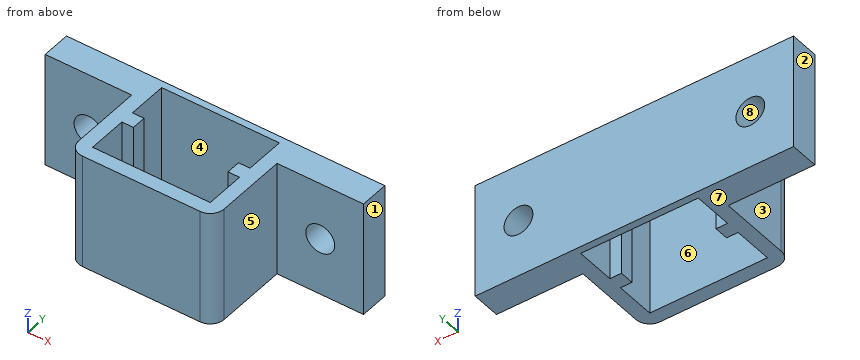
from build123d import *

# Parameters (mm, degrees)
F0_W     = 16.002
F0_H     = 12.5984
F1_DEPTH = 12.7
F2_W     = 9.525
F2_H     = 12.7
F3_DEPTH = 3.175
F4_R     = 1.524
F5_R     = 1.5875
F6_DEPTH = 25.4


with BuildPart() as f1:
    # F0 (on Top) → F1 (new body)
    with BuildSketch(Plane.XY):
        with Locations((0, 4.7752)):
            Rectangle(F0_W, F0_H)
        Polygon((6.477, 4.3688), (6.477, 0), (-6.477, 0), (-6.477, 4.3688), (-5.207, 4.3688), (-5.207, 5.9436), (-6.477, 5.9436), (-6.477, 10.3124), (6.477, 10.3124), (6.477, 5.9436), (5.207, 5.9436), (5.207, 4.3688), align=None, mode=Mode.SUBTRACT)
    extrude(amount=F1_DEPTH)

    # F2 (on face) → F3 (join)
    with BuildSketch(Plane(origin=(0, 11.0744, 0), x_dir=(-1, 0, 0), z_dir=(0, 1, 0))):
        with Locations((12.7635, 6.35)):
            Rectangle(F2_W, F2_H)
        with Locations((-12.7635, 6.35)):
            Rectangle(F2_W, F2_H)
    extrude(amount=-F3_DEPTH)

    # F4
    f4_edges = [f1.edges().sort_by_distance(p)[0] for p in [
        (-8.001, -1.524, 6.35),
        (8.001, -1.524, 6.35),
    ]]
    fillet(f4_edges, radius=F4_R)

    # F5 (on face) → F6 (cut)
    with BuildSketch(Plane.XZ.offset(-7.8994)):
        with Locations((-12.7635, 6.35)):
            Circle(F5_R)
        with Locations((12.7635, 6.35)):
            Circle(F5_R)
    extrude(amount=-F6_DEPTH, mode=Mode.SUBTRACT)


solid = f1.part
Source: CAD feature listing. Evaluate the final solid. Frame: model axes, mm. Face numbers are marked on the shaded views. A direction names the side the tool comes from. Give positions to 0.01 mm unless a question says otherwise; leave off trailing zeros. Loops run counter-clockwise (first coordinate to the right, second up) from the corner with the lowest first, then second, coordinate; pieces in that order, holes last. Notation, with made-up numbers: (69, -7.5) -> (76, -7.5) arc R25 ccw to (76, 6.5) -> close; hole circle Ø6 at (0.5, 81.5). An arc over 180 degrees is marked (long way). Use a Markdown table: item, result. Add a question column.
1) Section query C-C, the plane x = -6. Return the cut outline in (y, z), then the cut area to 3 significant figures.
2) Section query A-A, the plane z = 6.35. Count the separate pieces of the cut face and the enclosed holes in it, then the cut area to 3 significant figures.
3) Section query B-B, the plane y = 1.25. Return the cut outline in (x, z), then the cut area to 3 significant figures.
4) First-contact query: pin 1 (1.5 mm diameter, centred on y = 6, z = 10, fed in from -X); pin 2 (5 mm diameter, centred on x = 11, z = 9, fed in from -Y); pin 3 (2.5 mm diameter, centred on x = 12.76, z = 6.35, fed in from +Y); pin 4 (1.3 mm diameter, centred on y = 5.5, z = 8, fed in from +X). Flat tips, straight axial feed; report the tip coordinate or a pass-through.
5) Reachability of the marked faces 1, 2, 3, 4 and 5 from +Z, -Z, +X, -X, +Y, -Y: full face, straight path, thin tool, end or side. Return the list, or none.
6) Line query: line 1 along Y through (x, z) = (3, 2.5); line 2 along X through (y, z) = (9.75, 9.5); line 3 along X through (y, z) = (4, 8.5). Output: solid intervals per line, ascending. Write a range as [from, to].
7) Section query D-D, the plane z = 2.25. Return the cut outline in (x, y), then the cut area to 4 significant figures.
8) Pull-direction query (Z, two-part tool) for the marked faces 6, 7 and 8; classes: +Z half, -Z half, draft (parallel to the pull), parting line (faces both ways), or undercut.
Numbers:
| question | item | result |
|---|---|---|
| 1 | outline | (-1.52, 0) -> (0, 0) -> (0, 12.7) -> (-1.52, 12.7) -> close; (4.37, 0) -> (5.94, 0) -> (5.94, 12.7) -> (4.37, 12.7) -> close; (10.31, 0) -> (11.07, 0) -> (11.07, 12.7) -> (10.31, 12.7) -> close |
| 1 | area | 49.0 mm2 |
| 2 | separate pieces | 3 |
| 2 | enclosed holes | 1 |
| 2 | area | 111 mm2 |
| 3 | outline | (-8, 0) -> (-6.48, 0) -> (-6.48, 12.7) -> (-8, 12.7) -> close; (6.48, 0) -> (8, 0) -> (8, 12.7) -> (6.48, 12.7) -> close |
| 3 | area | 38.7 mm2 |
| 4 | pin 1 | stops at x = -8 |
| 4 | pin 2 | stops at y = 7.9 |
| 4 | pin 3 | passes through |
| 4 | pin 4 | stops at x = 8 |
| 5 | face 1 | +Z, -Z, +X, +Y, -Y |
| 5 | face 2 | +Z, -Z, -X, +Y, -Y |
| 5 | face 3 | +Z, -Z, -X, -Y |
| 5 | face 4 | +Z, -Z |
| 5 | face 5 | +Z, -Z, +X, -Y |
| 6 | line 1 | y = [-1.52, 0], [10.31, 11.07] |
| 6 | line 2 | x = [-17.53, -6.48], [6.48, 17.53] |
| 6 | line 3 | x = [-8, -6.48], [6.48, 8] |
| 7 | outline | (-17.53, 7.9) -> (-8, 7.9) -> (-8, 0) arc R1.52 ccw to (-6.48, -1.52) -> (6.48, -1.52) arc R1.52 ccw to (8, 0) -> (8, 7.9) -> (17.53, 7.9) -> (17.53, 11.07) -> (-17.53, 11.07) -> close; hole (-6.48, 0) -> (6.48, 0) -> (6.48, 4.37) -> (5.21, 4.37) -> (5.21, 5.94) -> (6.48, 5.94) -> (6.48, 10.31) -> (-6.48, 10.31) -> (-6.48, 5.94) -> (-5.21, 5.94) -> (-5.21, 4.37) -> (-6.48, 4.37) -> close |
| 7 | area | 131.5 mm2 |
| 8 | face 6 | draft |
| 8 | face 7 | -Z half |
| 8 | face 8 | undercut |
